Input: part model. Units: mm. Frame: model coordinates. A direction names the side the tool comes from. Coordinates: 2 decimals unless noted, no trailing zeros. Order: outer loops, then holes, each group sorted by start corner. A loop starts at its lowest first (then second) coordinate and runs counter-clockwise, first axis right, second up. Notation, with made-up numbers: M 86.5,85 L 122.5,85 A24 ccw 122.5,118 Z; hole C 39,37.25 d4. An arc over 180 degrees is marked long. One line per item, written item: value.
```python
from build123d import *

# Parameters (mm, degrees)
SKETCH1_W                      = 98
SKETCH1_H                      = 45
BOSS_EXTRUDE1_DEPTH            = 10
CONVERT_SOLID1_START           = 1.5
CONVERT_SOLID1_OUTLINE_W       = 98
CONVERT_SOLID1_OUTLINE_H       = 45
CONVERT_SOLID1_DEPTH           = 8.5
EDGE_FLANGE1_STRIP_W           = 14
EDGE_FLANGE1_STRIP_H           = 1.5
EDGE_FLANGE1_STRIP_CUT_DEPTH   = 98
EDGE_FLANGE1_DEPTH             = 98
EDGE_FLANGE2_STRIP_W           = 14
EDGE_FLANGE2_STRIP_H           = 1.5
EDGE_FLANGE2_STRIP_CUT_DEPTH   = 36
EDGE_FLANGE2_STRIP_2_W         = 14
EDGE_FLANGE2_STRIP_2_H         = 1.5
EDGE_FLANGE2_STRIP_CUT_2_DEPTH = 36
EDGE_FLANGE2_DEPTH             = 36
EDGE_FLANGE2_BEND_DEPTH        = 36
SKETCH17_W                     = 5.5
SKETCH17_H                     = 5.5
CUT_EXTRUDE1_DEPTH             = 79.41077732
SKETCH18_W                     = 1.5
SKETCH18_H                     = 39.5
BOSS_EXTRUDE2_DEPTH            = 7.3
EDGE_FLANGE3_STRIP_W           = 14
EDGE_FLANGE3_STRIP_H           = 1.5
EDGE_FLANGE3_STRIP_CUT_DEPTH   = 39.5
EDGE_FLANGE3_STRIP_2_W         = 14
EDGE_FLANGE3_STRIP_2_H         = 1.5
EDGE_FLANGE3_STRIP_CUT_2_DEPTH = 39.5
EDGE_FLANGE3_DEPTH             = 39.5
EDGE_FLANGE3_BEND_DEPTH        = 39.5
SKETCH25_R                     = 2.15
CUT_EXTRUDE2_DEPTH             = 70.153018734
SKETCH26_R                     = 3
CUT_EXTRUDE3_DEPTH             = 10


# Read off the part's stored shape, not the designer's step: Convert-Solid1
# Sheet-metal steps are written as plain solids
with BuildPart() as part:
    # Sketch1 → Boss-Extrude1 (new body)
    with BuildSketch(Plane.XY):
        Rectangle(SKETCH1_W, SKETCH1_H)
    extrude(amount=BOSS_EXTRUDE1_DEPTH)

    # Convert-Solid1 outline → Convert-Solid1 (cut)
    with BuildSketch(Plane.XY.offset(CONVERT_SOLID1_START)):
        Rectangle(CONVERT_SOLID1_OUTLINE_W, CONVERT_SOLID1_OUTLINE_H)
    extrude(amount=CONVERT_SOLID1_DEPTH, mode=Mode.SUBTRACT)

    # Edge-Flange1 strip (across the edge) → Edge-Flange1 strip cut (cut)
    with BuildSketch(Plane(origin=(-49, -22.5, 1.5), x_dir=(0, 1, 0), z_dir=(1, 0, 0))):
        with Locations((-1.5, -0.75)):
            Rectangle(EDGE_FLANGE1_STRIP_W, EDGE_FLANGE1_STRIP_H)
    extrude(amount=EDGE_FLANGE1_STRIP_CUT_DEPTH, mode=Mode.SUBTRACT)

    # Edge-Flange1 section (across the edge) → Edge-Flange1 (add)
    with BuildSketch(Plane(origin=(-49, -22.5, 1.5), x_dir=(0, 1, 0), z_dir=(1, 0, 0))):
        with BuildLine():
            Line((0, 4), (0, 40))
            Line((0, 40), (1.5, 40))
            Line((1.5, 40), (1.5, 4))
            ThreePointArc((1.5, 4), (2.671572875, 1.171572875), (5.5, 0))
            Line((5.5, 0), (5.5, -1.5))
            ThreePointArc((5.5, -1.5), (1.610912703, 0.110912703), (0, 4))
        make_face()
    extrude(amount=EDGE_FLANGE1_DEPTH)

    # Edge-Flange2 strip (across the edge) → Edge-Flange2 strip cut (cut)
    with BuildSketch(Plane(origin=(49, -21, 41.5), x_dir=(-1, 0, 0), z_dir=(0, 0, -1))):
        with Locations((-1.5, -0.75)):
            Rectangle(EDGE_FLANGE2_STRIP_W, EDGE_FLANGE2_STRIP_H)
    extrude(amount=EDGE_FLANGE2_STRIP_CUT_DEPTH, mode=Mode.SUBTRACT)

    # Edge-Flange2 strip 2 (across the edge) → Edge-Flange2 strip cut 2 (cut)
    with BuildSketch(Plane(origin=(-49, -21, 5.5), x_dir=(1, 0, 0), z_dir=(0, 0, 1))):
        with Locations((-1.5, -0.75)):
            Rectangle(EDGE_FLANGE2_STRIP_2_W, EDGE_FLANGE2_STRIP_2_H)
    extrude(amount=EDGE_FLANGE2_STRIP_CUT_2_DEPTH, mode=Mode.SUBTRACT)

    # Edge-Flange2 section (across the edge) → Edge-Flange2 (add)
    with BuildSketch(Plane(origin=(49, -21, 41.5), x_dir=(-1, 0, 0), z_dir=(0, 0, -1))):
        with BuildLine():
            Line((0, 4), (0, 43.5))
            Line((0, 43.5), (1.5, 43.5))
            Line((1.5, 43.5), (1.5, 4))
            ThreePointArc((1.5, 4), (2.671572875, 1.171572875), (5.5, 0))
            Line((5.5, 0), (5.5, -1.5))
            ThreePointArc((5.5, -1.5), (1.610912703, 0.110912703), (0, 4))
        make_face()
    extrude(amount=EDGE_FLANGE2_DEPTH)

    # Edge-Flange2 section 2 (across the edge) → Edge-Flange2 bend (add)
    with BuildSketch(Plane(origin=(-49, -21, 5.5), x_dir=(1, 0, 0), z_dir=(0, 0, 1))):
        with BuildLine():
            Line((0, 4), (0, 43.5))
            Line((0, 43.5), (1.5, 43.5))
            Line((1.5, 43.5), (1.5, 4))
            ThreePointArc((1.5, 4), (2.671572875, 1.171572875), (5.5, 0))
            Line((5.5, 0), (5.5, -1.5))
            ThreePointArc((5.5, -1.5), (1.610912703, 0.110912703), (0, 4))
        make_face()
    extrude(amount=EDGE_FLANGE2_BEND_DEPTH)

    # Sketch17 → Cut-Extrude1 (cut, through all)
    with BuildSketch(Plane(origin=(0, 22.5, 0), x_dir=(1, 0, 0), z_dir=(0, 1, 0))):
        with Locations((-46.25, -2.75)):
            Rectangle(SKETCH17_W, SKETCH17_H)
        with Locations((46.25, -2.75)):
            Rectangle(SKETCH17_W, SKETCH17_H)
    extrude(amount=-CUT_EXTRUDE1_DEPTH, mode=Mode.SUBTRACT)

    # Sketch18 → Boss-Extrude2 (add)
    with BuildSketch(Plane(origin=(0, 0, 5.5), x_dir=(-1, 0, 0), z_dir=(0, 0, -1))):
        with Locations((-48.25, 2.75)):
            Rectangle(SKETCH18_W, SKETCH18_H)
        with Locations((48.25, 2.75)):
            Rectangle(SKETCH18_W, SKETCH18_H)
    extrude(amount=BOSS_EXTRUDE2_DEPTH)

    # Edge-Flange3 strip (across the edge) → Edge-Flange3 strip cut (cut)
    with BuildSketch(Plane(origin=(47.5, 22.5, -1.8), x_dir=(0, 0, 1), z_dir=(0, -1, 0))):
        with Locations((-1.5, -0.75)):
            Rectangle(EDGE_FLANGE3_STRIP_W, EDGE_FLANGE3_STRIP_H)
    extrude(amount=EDGE_FLANGE3_STRIP_CUT_DEPTH, mode=Mode.SUBTRACT)

    # Edge-Flange3 strip 2 (across the edge) → Edge-Flange3 strip cut 2 (cut)
    with BuildSketch(Plane(origin=(-47.5, -17, -1.8), x_dir=(0, 0, 1), z_dir=(0, 1, 0))):
        with Locations((-1.5, -0.75)):
            Rectangle(EDGE_FLANGE3_STRIP_2_W, EDGE_FLANGE3_STRIP_2_H)
    extrude(amount=EDGE_FLANGE3_STRIP_CUT_2_DEPTH, mode=Mode.SUBTRACT)

    # Edge-Flange3 section (across the edge) → Edge-Flange3 (add)
    with BuildSketch(Plane(origin=(47.5, 22.5, -1.8), x_dir=(0, 0, 1), z_dir=(0, -1, 0))):
        with BuildLine():
            Line((0, 4), (0, 14))
            Line((0, 14), (1.5, 14))
            Line((1.5, 14), (1.5, 4))
            ThreePointArc((1.5, 4), (2.671572875, 1.171572875), (5.5, 0))
            Line((5.5, 0), (5.5, -1.5))
            ThreePointArc((5.5, -1.5), (1.610912703, 0.110912703), (0, 4))
        make_face()
    extrude(amount=EDGE_FLANGE3_DEPTH)

    # Edge-Flange3 section 2 (across the edge) → Edge-Flange3 bend (add)
    with BuildSketch(Plane(origin=(-47.5, -17, -1.8), x_dir=(0, 0, 1), z_dir=(0, 1, 0))):
        with BuildLine():
            Line((0, 4), (0, 14))
            Line((0, 14), (1.5, 14))
            Line((1.5, 14), (1.5, 4))
            ThreePointArc((1.5, 4), (2.671572875, 1.171572875), (5.5, 0))
            Line((5.5, 0), (5.5, -1.5))
            ThreePointArc((5.5, -1.5), (1.610912703, 0.110912703), (0, 4))
        make_face()
    extrude(amount=EDGE_FLANGE3_BEND_DEPTH)

    # Sketch25 → Cut-Extrude2 (cut, through all)
    with BuildSketch(Plane(origin=(0, 0, -1.8), x_dir=(-1, 0, 0), z_dir=(0, 0, -1))):
        with Locations((38.5, 15.5)):
            Circle(SKETCH25_R)
        with Locations((38.5, -10)):
            Circle(SKETCH25_R)
        with Locations(Location((-38.5, -10, 0), (0, 0, 180))):
            Circle(SKETCH25_R)
        with Locations(Location((-38.5, 15.5, 0), (0, 0, 180))):
            Circle(SKETCH25_R)
    extrude(amount=-CUT_EXTRUDE2_DEPTH, mode=Mode.SUBTRACT)

    # Sketch26 → Cut-Extrude3 (cut)
    with BuildSketch(Plane.XY.offset(1.5)):
        with Locations((0, 11.25)):
            Circle(SKETCH26_R)
        with Locations((0, -5.75)):
            Circle(SKETCH26_R)
    extrude(amount=-CUT_EXTRUDE3_DEPTH, mode=Mode.SUBTRACT)


solid = part.part
```
(1) First-contact query: pin 1 (10 mm diameter, centred on x = 1, y = 7.5, fed in from +Z); pin 2 (5 mm diameter, centred on x = 19.5, y = 6, fed in from -Z); pin 3 (11 mm diameter, centred on x = 20.5, z = 25, fed in from +Y). Flat tips, straight axial feed; report the tip coordinate or a pass-through.
Data:
pin 1: stops at z = 1.5
pin 2: stops at z = 0
pin 3: stops at y = -21
(2) Cut plane A-A on x = 0. Output: boundary loops of the cut face in (y, z), plus the area to 3 significant figures.
Data:
outline: M -22.5,5.5 A5.5 ccw -17,0 L -8.75,0 L -8.75,1.5 L -17,1.5 A4 cw -21,5.5 L -21,41.5 L -22.5,41.5 Z; M -2.75,0 L 8.25,0 L 8.25,1.5 L -2.75,1.5 Z; M 14.25,0 L 22.5,0 L 22.5,1.5 L 14.25,1.5 Z
area: 106 mm2
(3) Access query for faces 4 (the flat face through (-48, 22.5, 17)), 5 (the flat face through (-46.4, -20.1, 5.5)), 6 (the flat face through (-1, -21, 24)). Directions: +Z, -Z, +X, -X, +Y, -Y. A direction counts if a zero-diameter tool reaches every point of the face in a straight line with its end or side. Return the directions, or none.
Data:
face 4: +Z, -Z, +X, -X, +Y
face 5: -Z, -X, -Y
face 6: +Z, +Y
(4) Cut plane B-B on y = -5.75. Output: boundary loops of the cut face in (x, z).
Data:
outline: M -49,3.7 A5.5 ccw -43.5,-1.8 L -33.5,-1.8 L -33.5,-0.3 L -43.5,-0.3 A4 cw -47.5,3.7 L -47.5,41.5 L -49,41.5 Z; M -43.5,0 L -3,0 L -3,1.5 L -43.5,1.5 Z; M 3,0 L 43.5,0 L 43.5,1.5 L 3,1.5 Z; M 33.5,-1.8 L 43.5,-1.8 A5.5 ccw 49,3.7 L 49,41.5 L 47.5,41.5 L 47.5,3.7 A4 cw 43.5,-0.3 L 33.5,-0.3 Z
(5) Ray query, line 1 (Y direction, x = -38.5, z = -1); line 2 (X direction, y = 18.5, z = 27); line 3 (Y direction, x = 0, z = 0.55). Return the intervals inside material, ascending. Write a range as from..to.
Data:
line 1: y = -17..-12.15, -7.85..13.35, 17.65..22.5
line 2: x = -49..-47.5, 47.5..49
line 3: y = -19.4..-8.75, -2.75..8.25, 14.25..22.5
(6) Draft query along Y for faces 1 (the flat face through (-43.5, -2, 1)), 2 (the cylindrical face through (47.35, -20.93, 23.75)), 3 (the cylindrical face through (40.55, -10.65, 0.74)). Return one class per face: released by +Y, released by -Y, zero draft, split by the parting line, or undercut.
Data:
face 1: zero draft
face 2: released by -Y
face 3: undercut
(7) Cut plane C-C on z = 26. Output: boundary loops of the cut face in (x, y).
Data:
outline: M -49,-17 A5.5 ccw -43.5,-22.5 L 43.5,-22.5 A5.5 ccw 49,-17 L 49,22.5 L 47.5,22.5 L 47.5,-17 A4 cw 43.5,-21 L -43.5,-21 A4 cw -47.5,-17 L -47.5,22.5 L -49,22.5 Z
(8) Cut plane D-D on y = 0. Output: boundary loops of the cut face in (x, z), plus the area to 3 significant figures.
Data:
outline: M -49,3.7 A5.5 ccw -43.5,-1.8 L -33.5,-1.8 L -33.5,-0.3 L -43.5,-0.3 A4 cw -47.5,3.7 L -47.5,41.5 L -49,41.5 Z; M -43.5,0 L 43.5,0 L 43.5,1.5 L -43.5,1.5 Z; M 33.5,-1.8 L 43.5,-1.8 A5.5 ccw 49,3.7 L 49,41.5 L 47.5,41.5 L 47.5,3.7 A4 cw 43.5,-0.3 L 33.5,-0.3 Z
area: 296 mm2
